The listing builds one solid part. Answer for the finished solid, in the listing's coordinates (mm). Face numbers are marked on the shaded views. A direction names the side the tool comes from. Round coordinates to 2 decimals unless told otherwise and drop trailing zeros. Loops run counter-clockwise (first coordinate to the right, second up) from the corner with the lowest first, then second, coordinate; pieces in that order, holes last. Notation, with made-up numbers: (88, 1.5) -> (141, 1.5) arc R16 cw to (141, 27.5) -> close; hole circle Ø8 at (-35.5, -27). An arc over 180 degrees is marked (long way). Use a Markdown table: item, result. Add a question column.
Q1. Section A-A on z = 0 is taken. Give the vertices of the cut face in (x, y).
Q2. Consider line 1 (X direction, y = 0.2, z = 0); line 2 (X direction, y = 4.7, z = 0); line 3 (X direction, y = 2.1, z = 0). Determine where each line is inside the solid, lowest interval first.
Q3. Given pin 1 Ø1 at (y, z) = (1.5, 5) entering from +X; pin 2 Ø4 at (x, z) = (2.5, -0.5) entering from +Y; pin 3 Ø1 at (y, z) = (1.5, -4) entering from +X; pin 4 Ø6.5 at (x, z) = (0, 0) entering from -Y, each flat-ended and moving along its own axis, determine where each tip first touches the part or whether it passes through.
Q4. Section C-C on y = 2.55 is taken. Give the vertices of the cut face in (x, z).
Q5. Section B-B on x = 0 is taken. Give the vertices of the cut face in (y, z).
Q6. Which of the six approach directions +Z, -Z, +X, -X, +Y, -Y give full straight-line access (tool end or side, diameter ignored) to the marked faces 4 and 5?
Q7. For a pull along X with two mould halves and no side action, classify the marked faces 1, 2 and 3 as released by +X, released by -X, zero draft, split by the parting line, or undercut.
Q8. Section D-D on z = 4.5 is taken. Give the vertices of the cut face in (x, y), then the cut area to 3 significant figures.
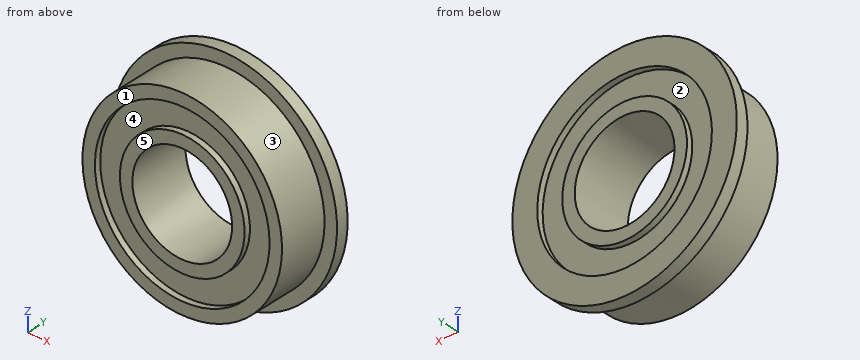
from build123d import *

# Parameters (mm, degrees)
SKETCH1_R           = 8
SKETCH1_R_2         = 4
BOSS_EXTRUDE1_DEPTH = 4
SKETCH2_R           = 9
SKETCH2_R_2         = 4
BOSS_EXTRUDE2_DEPTH = 1
SKETCH3_R           = 7
SKETCH3_R_2         = 5
CUT_EXTRUDE1_DEPTH  = 0.5
CUT_EXTRUDE2_START  = -0.5
SKETCH4_R           = 7
SKETCH4_R_2         = 5
CUT_EXTRUDE2_DEPTH  = 0.5


with BuildPart() as part:
    # Sketch1 → Boss-Extrude1 (new body)
    with BuildSketch(Plane(origin=(0, 0, 0), x_dir=(1, 0, 0), z_dir=(0, 1, 0))):
        with Locations(Location((0, 0, 0), (0, 0, 270))):
            Circle(SKETCH1_R)
        with Locations(Location((0, 0, 0), (0, 0, 270))):
            Circle(SKETCH1_R_2, mode=Mode.SUBTRACT)
    extrude(amount=BOSS_EXTRUDE1_DEPTH)

    # Sketch2 → Boss-Extrude2 (add)
    with BuildSketch(Plane(origin=(0, 4, 0), x_dir=(1, 0, 0), z_dir=(0, 1, 0))):
        with Locations(Location((0, 0, 0), (0, 0, 270))):
            Circle(SKETCH2_R)
        with Locations(Location((0, 0, 0), (0, 0, 270))):
            Circle(SKETCH2_R_2, mode=Mode.SUBTRACT)
    extrude(amount=BOSS_EXTRUDE2_DEPTH)

    # Sketch3 → Cut-Extrude1 (cut)
    with BuildSketch(Plane.XZ):
        with Locations(Location((0, 0, 0), (0, 0, 270))):
            Circle(SKETCH3_R)
        with Locations(Location((0, 0, 0), (0, 0, 270))):
            Circle(SKETCH3_R_2, mode=Mode.SUBTRACT)
    extrude(amount=-CUT_EXTRUDE1_DEPTH, mode=Mode.SUBTRACT)

    # Sketch4 → Cut-Extrude2 (cut)
    with BuildSketch(Plane(origin=(0, 5, 0), x_dir=(1, 0, 0), z_dir=(0, 1, 0)).offset(CUT_EXTRUDE2_START)):
        with Locations(Location((0, 0, 0), (0, 0, 90))):
            Circle(SKETCH4_R)
        with Locations(Location((0, 0, 0), (0, 0, 90))):
            Circle(SKETCH4_R_2, mode=Mode.SUBTRACT)
    extrude(amount=CUT_EXTRUDE2_DEPTH, mode=Mode.SUBTRACT)


solid = part.part
Checked values:
| question | item | result |
|---|---|---|
| 1 | outline | (-9, 4) -> (-8, 4) -> (-8, 0) -> (-7, 0) -> (-7, 0.5) -> (-5, 0.5) -> (-5, 0) -> (-4, 0) -> (-4, 5) -> (-5, 5) -> (-5, 4.5) -> (-7, 4.5) -> (-7, 5) -> (-9, 5) -> close; (4, 0) -> (5, 0) -> (5, 0.5) -> (7, 0.5) -> (7, 0) -> (8, 0) -> (8, 4) -> (9, 4) -> (9, 5) -> (7, 5) -> (7, 4.5) -> (5, 4.5) -> (5, 5) -> (4, 5) -> close |
| 2 | line 1 | x = -8 to -7, -5 to -4, 4 to 5, 7 to 8 |
| 2 | line 2 | x = -9 to -7, -5 to -4, 4 to 5, 7 to 9 |
| 2 | line 3 | x = -8 to -4, 4 to 8 |
| 3 | pin 1 | stops at x = 6.61 |
| 3 | pin 2 | stops at y = 5 |
| 3 | pin 3 | stops at x = 7.19 |
| 3 | pin 4 | passes through |
| 4 | outline | circle Ø16 at (0, 0); hole circle Ø8 at (0, 0) |
| 5 | outline | (0, -8) -> (4, -8) -> (4, -9) -> (5, -9) -> (5, -7) -> (4.5, -7) -> (4.5, -5) -> (5, -5) -> (5, -4) -> (0, -4) -> (0, -5) -> (0.5, -5) -> (0.5, -7) -> (0, -7) -> close; (0, 4) -> (5, 4) -> (5, 5) -> (4.5, 5) -> (4.5, 7) -> (5, 7) -> (5, 9) -> (4, 9) -> (4, 8) -> (0, 8) -> (0, 7) -> (0.5, 7) -> (0.5, 5) -> (0, 5) -> close |
| 6 | face 4 | -Y |
| 6 | face 5 | +Z, -Z, +X, -X, -Y |
| 7 | face 1 | zero draft |
| 7 | face 2 | undercut |
| 7 | face 3 | split by the parting line |
| 8 | outline | (-7.79, 4) -> (-6.61, 4) -> (-6.61, 0) -> (-5.36, 0) -> (-5.36, 0.5) -> (-2.18, 0.5) -> (-2.18, 0) -> (2.18, 0) -> (2.18, 0.5) -> (5.36, 0.5) -> (5.36, 0) -> (6.61, 0) -> (6.61, 4) -> (7.79, 4) -> (7.79, 5) -> (5.36, 5) -> (5.36, 4.5) -> (2.18, 4.5) -> (2.18, 5) -> (-2.18, 5) -> (-2.18, 4.5) -> (-5.36, 4.5) -> (-5.36, 5) -> (-7.79, 5) -> close |
| 8 | area | 62.1 mm2 |
